Source: three-view drawing plus pictorial views. Frame: mm from the lowest corner of the part. Coordinates: 2 decimals unless noted, no trailing zeros. Loops run counter-clockwise (first coordinate to the right, second up) from the corner with the lowest first, then second, coordinate; pieces in that order, holes last.
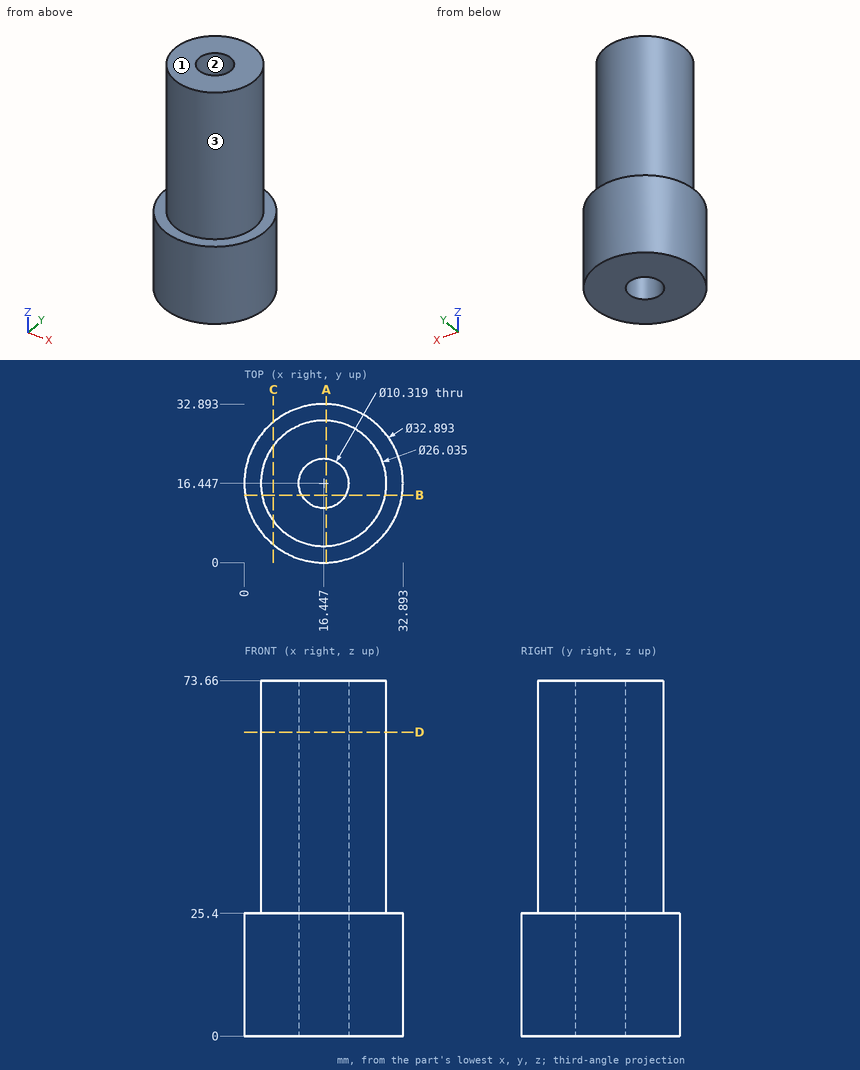
Q1. Line query: line 1 along X through (y, z) = (16.5, 19) (1 decimal); line 2 along Z through (x, y) = (2.5, 13.5); line 3 along Y through (x, z) = (17, 50) (1 decimal). Output: solid intervals per line, ascending.
Q2. Contact query for flat-ended pins moving along their axis: pin 1 Ø3 at (y, z) = (4.5, 56.5) entering from -X; pin 2 Ø4 at (x, z) = (13.5, 27) entering from -Y; pin 3 Ø5 at (x, z) = (8.5, 31) entering from +Y; pin 4 Ø9.5 at (x, y) = (16.45, 16.45) entering from -Z. Output: stop coordinate, or through.
Q3. Draft query along Y for the marked faces 1, 2 and 3. Return one class per face: +Y half, -Y half, draft (parallel to the pull), parting line (faces both ways), or undercut.
Q4. Section C-C, the plane x = 6. Return the cut outline in (y, z), plus the area to 4 significant figures.
Q5. Section B-B, the plane y = 14. Return the cut outline in (x, z) (1 decimal).
Q6. Section A-A, the plane x = 17. Return the cut outline in (y, z).
Q7. Section D-D, the plane z = 63. Return the cut outline in (x, y) (1 decimal).
Derived:
1. line 1: x = 0 to 11.3, 21.6 to 32.9
1. line 2: z = 0 to 25.4
1. line 3: y = 3.4 to 11.3, 21.6 to 29.5
2. pin 1: stops at x = 8.68
2. pin 2: stops at y = 0.09
2. pin 3: stops at y = 28.27
2. pin 4: passes through
3. face 1: draft
3. face 2: undercut
3. face 3: parting line
4. outline: (3.74, 0) - (29.15, 0) - (29.15, 25.4) - (24.21, 25.4) - (24.21, 73.66) - (8.68, 73.66) - (8.68, 25.4) - (3.74, 25.4) - close
4. area: 1,395 mm2
5. outline: (0.2, 0) - (11.9, 0) - (11.9, 73.7) - (3.7, 73.7) - (3.7, 25.4) - (0.2, 25.4) - close; (21, 0) - (32.7, 0) - (32.7, 25.4) - (29.2, 25.4) - (29.2, 73.7) - (21, 73.7) - close
6. outline: (0.01, 0) - (11.32, 0) - (11.32, 73.66) - (3.44, 73.66) - (3.44, 25.4) - (0.01, 25.4) - close; (21.58, 0) - (32.88, 0) - (32.88, 25.4) - (29.45, 25.4) - (29.45, 73.66) - (21.58, 73.66) - close
7. outline: circle Ø26 at (16.4, 16.4); hole circle Ø10.3 at (16.4, 16.4)
